Check sheet for the modelled part. Datum: model origin and axes. Units: mm. Face numbers are marked on the shaded views. A direction names the side the tool comes from. Round coordinates to 2 decimals unless told otherwise and drop trailing zeros. Loops run counter-clockwise (first coordinate to the right, second up) from the corner with the lowest first, then second, coordinate; pieces in that order, holes last. Notation, with made-up numbers: (73, 13) -> (96, 13) arc R32 cw to (96, 43) -> close; hole circle Ø7 at (-33, -29). An arc over 180 degrees is marked (long way). One line per item, written item: value. Start each with the question number.
1. Release check for a two-part mould opening along X. For the marked faces 1, 2 and 3 record: +X half, -X half, draft (parallel to the pull), parting line (faces both ways), or undercut.
2. Set-up check for the marked faces 4, 5, 6 and 7: record each of +Z, -Z, +X, -X, +Y, -Y from which the full face is reachable in a straight line by a thin tool's end or side.
3. Material ranges on L1, parallel to Y at x = 7, z = 19.5; L2, parallel to X at y = -1.5, z = 21; L3, parallel to Z at x = -14, y = 9.5, recorded low to high.
4. Go/stop test with flat-tipped pins: pin 1 (2.5 mm diameter, centred on y = 2.5, z = -6.5, fed in from -X); pin 2 (10 mm diameter, centred on x = 17.5, y = 3.5, fed in from +Z); pin 3 (11 mm diameter, centred on y = -5, z = -17.5, fed in from +X). Record where each tip stops, or that it passes through.
5. Cross-section at B-B on y = -25. Record the cut outline in (x, z).
6. Cross-section at A-A on x = 0. Record the cut outline in (y, z), then the cut area to 3 significant figures.
7. Cross-section at C-C on y = 6. Count the separate pieces of the cut face and the enclosed holes in it, then the cut area to 3 significant figures.
from build123d import *
from build123d.topology import SkipClean

# Parameters (mm, degrees)
HINGE_DEPTH           = 8.89
HINGE_2_DEPTH         = 8.89
SKETCH2_R             = 2.54
HINGE_HOLES_DEPTH     = 50.270844447
BODY_START            = 12.7
BODY_DEPTH            = 12.7
BOTTOM_PLATE_START    = 5.08
BOTTOM_PLATE_DEPTH    = 5.08
TUBE_CONNECTION_DEPTH = 19.05
BACKSTOP_DEPTH        = 2.921
CONNECT_TO_BASE_START = 12.7
CONNECT_TO_BASE_DEPTH = 12.7
SKETCH13_R            = 7.62
BOLT_ACCESS_DEPTH     = 21.59
BOTTOM_CHAMFER_SIZE   = 1.27


with BuildPart() as part:
    # Sketch1 → hinge (new body)
    with BuildSketch(Plane(origin=(0, 0, 0), x_dir=(1, 0, 0), z_dir=(0, 1, 0))):
        with BuildLine():
            ThreePointArc((-6.35, 26.882708313), (-9.597376484, 25.901599774), (-12.7, 24.529828908))
            Line((-12.7, 24.529828908), (-12.7, 11.829828908))
            Line((-12.7, 11.829828908), (-24.961122857, 11.829828908))
            ThreePointArc((-24.961122857, 11.829828908), (-26.9489436, 6.062750619), (-27.6225, 0))
            Line((-27.6225, 0), (-25.0825, 0))
            ThreePointArc((-25.0825, 0), (-24.632521559, 4.729766155), (-23.298731406, 9.289828908))
            Line((-23.298731406, 9.289828908), (-12.7, 9.289828908))
            Line((-12.7, 9.289828908), (-12.7, 0))
            Line((-12.7, 0), (-6.35, 0))
            Line((-6.35, 0), (-6.35, 26.882708313))
        make_face()
    hinge = extrude(amount=HINGE_DEPTH)


with BuildPart() as body_2:
    # Sketch1 → hinge 2 (new body)
    with BuildSketch(Plane(origin=(0, 0, 0), x_dir=(1, 0, 0), z_dir=(0, 1, 0))):
        with BuildLine():
            ThreePointArc((12.7, 24.529828908), (9.597376484, 25.901599774), (6.35, 26.882708313))
            Line((6.35, 26.882708313), (6.35, 0))
            Line((6.35, 0), (12.7, 0))
            Line((12.7, 0), (12.7, 9.289828908))
            Line((12.7, 9.289828908), (23.298731406, 9.289828908))
            ThreePointArc((23.298731406, 9.289828908), (24.632521559, 4.729766155), (25.0825, 0))
            Line((25.0825, 0), (27.6225, 0))
            ThreePointArc((27.6225, 0), (26.9489436, 6.062750619), (24.961122857, 11.829828908))
            Line((24.961122857, 11.829828908), (12.7, 11.829828908))
            Line((12.7, 11.829828908), (12.7, 24.529828908))
        make_face()
    hinge_2 = extrude(amount=HINGE_2_DEPTH)


with BuildPart() as hinge_holes_tool:
    # Sketch2 → hinge_holes (new, through all)
    with BuildSketch(Plane(origin=(12.7, 0, 0), x_dir=(0, 0, -1), z_dir=(1, 0, 0))):
        with Locations((19.262708313, 4.445)):
            Circle(SKETCH2_R)
    hinge_holes = extrude(amount=-HINGE_HOLES_DEPTH)


with BuildPart() as part_1:
    add(part.part)

    # hinge_holes: cut by hinge_holes_tool
    add(hinge_holes_tool.part, mode=Mode.SUBTRACT)



with BuildPart() as body_2_1:
    add(body_2.part)

    # hinge_holes: cut by hinge_holes_tool
    add(hinge_holes_tool.part, mode=Mode.SUBTRACT)


with BuildPart() as part_2:
    add(part_1.part)

    add(body_2_1.part)  # body merges body 2
    # Sketch5 → body (add)
    with BuildSketch(Plane.XZ.offset(BODY_START)):
        with BuildLine():
            Line((-27.6225, 0), (-25.0825, 0))
            ThreePointArc((-25.0825, 0), (-19.854542065, -15.327392656), (-6.35, -24.265393181))
            Line((-6.35, -24.265393181), (-6.35, -26.882708313))
            ThreePointArc((-6.35, -26.882708313), (-21.661087014, -17.140589711), (-27.6225, 0))
        make_face()
        with BuildLine():
            Line((25.0825, 0), (27.6225, 0))
            ThreePointArc((27.6225, 0), (21.661087014, -17.140589711), (6.35, -26.882708313))
            Line((6.35, -26.882708313), (6.35, -24.265393181))
            ThreePointArc((6.35, -24.265393181), (19.854542065, -15.327392656), (25.0825, 0))
        make_face()
    body = extrude(amount=-BODY_DEPTH)

    # Sketch6 → bottom_plate (add)
    with SkipClean():  # the faces are left unmerged after this step: merging them gives an invalid solid
        with BuildSketch(Plane.XZ.offset(12.7).offset(BOTTOM_PLATE_START)):
            with BuildLine():
                Line((13.97, 0), (3.81, 0))
                ThreePointArc((3.81, 0), (0, -3.81), (-3.81, 0))
                Line((-3.81, 0), (-13.97, 0))
                ThreePointArc((-13.97, 0), (-17.78, -3.81), (-21.59, 0))
                Line((-21.59, 0), (-27.6225, 0))
                ThreePointArc((-27.6225, 0), (0, -27.6225), (27.6225, 0))
                Line((27.6225, 0), (21.59, 0))
                ThreePointArc((21.59, 0), (17.78, -3.81), (13.97, 0))
            make_face()
        bottom_plate = extrude(amount=-BOTTOM_PLATE_DEPTH)

    # Sketch7 → tube_connection (add)
    with SkipClean():  # the faces are left unmerged after this step: merging them gives an invalid solid
        with BuildSketch(Plane.XZ.offset(17.78)):
            with BuildLine():
                Line((-22.86, 0), (-25.4, 0))
                ThreePointArc((-25.4, 0), (0, -25.4), (25.4, 0))
                Line((25.4, 0), (22.86, 0))
                ThreePointArc((22.86, 0), (0, -22.86), (-22.86, 0))
            make_face()
        tube_connection = extrude(amount=TUBE_CONNECTION_DEPTH)

    # Sketch10 → backstop (add)
    with SkipClean():  # the faces are left unmerged after this step: merging them gives an invalid solid
        with BuildSketch(Plane(origin=(0, 8.89, 0), x_dir=(1, 0, 0), z_dir=(0, 1, 0))):
            with BuildLine():
                Line((-23.298731406, 9.289828908), (-6.35, 9.289828908))
                Line((-6.35, 9.289828908), (-6.35, 11.829828908))
                Line((-6.35, 11.829828908), (-24.961122857, 11.829828908))
                ThreePointArc((-24.961122857, 11.829828908), (-26.9489436, 6.062750619), (-27.6225, 0))
                Line((-27.6225, 0), (-25.0825, 0))
                ThreePointArc((-25.0825, 0), (-24.632521559, 4.729766155), (-23.298731406, 9.289828908))
            make_face()
            with BuildLine():
                Line((6.35, 11.829828908), (24.961122857, 11.829828908))
                ThreePointArc((24.961122857, 11.829828908), (26.9489436, 6.062750619), (27.6225, 0))
                Line((27.6225, 0), (25.0825, 0))
                ThreePointArc((25.0825, 0), (24.632521559, 4.729766155), (23.298731406, 9.289828908))
                Line((23.298731406, 9.289828908), (6.35, 9.289828908))
                Line((6.35, 9.289828908), (6.35, 11.829828908))
            make_face()
        backstop = extrude(amount=BACKSTOP_DEPTH)

    # Mirror1: hinge, hinge 2, hinge_holes, body, bottom_plate, tube_connection, backstop across plane
    with SkipClean():  # the faces are left unmerged after this step: merging them gives an invalid solid
        add(hinge.mirror(Plane(origin=(0, 8.89, 0), x_dir=(1, 0, 0), z_dir=(0, 0, 1))))
        add(hinge_2.mirror(Plane(origin=(0, 8.89, 0), x_dir=(1, 0, 0), z_dir=(0, 0, 1))))
        add(hinge_holes.mirror(Plane(origin=(0, 8.89, 0), x_dir=(1, 0, 0), z_dir=(0, 0, 1))), mode=Mode.SUBTRACT)
        add(body.mirror(Plane(origin=(0, 8.89, 0), x_dir=(1, 0, 0), z_dir=(0, 0, 1))))
        add(bottom_plate.mirror(Plane(origin=(0, 8.89, 0), x_dir=(1, 0, 0), z_dir=(0, 0, 1))))
        add(tube_connection.mirror(Plane(origin=(0, 8.89, 0), x_dir=(1, 0, 0), z_dir=(0, 0, 1))))
        add(backstop.mirror(Plane(origin=(0, 8.89, 0), x_dir=(1, 0, 0), z_dir=(0, 0, 1))))

    # Sketch12 → connect_to_base (add)
    with SkipClean():  # the faces are left unmerged after this step: merging them gives an invalid solid
        with BuildSketch(Plane.XZ.offset(CONNECT_TO_BASE_START)):
            with BuildLine():
                Line((-6.35, -24.265393181), (-6.35, 24.265393181))
                ThreePointArc((-6.35, 24.265393181), (-9.615737574, 23.166126071), (-12.7, 21.629651089))
                Line((-12.7, 21.629651089), (-12.7, 11.829828908))
                Line((-12.7, 11.829828908), (-22.117571165, 11.829828908))
                ThreePointArc((-22.117571165, 11.829828908), (-22.743637238, 10.576330717), (-23.298731406, 9.289828908))
                Line((-23.298731406, 9.289828908), (-12.7, 9.289828908))
                Line((-12.7, 9.289828908), (-12.7, -9.289828908))
                Line((-12.7, -9.289828908), (-23.298731406, -9.289828908))
                ThreePointArc((-23.298731406, -9.289828908), (-22.743637238, -10.576330717), (-22.117571165, -11.829828908))
                Line((-22.117571165, -11.829828908), (-12.7, -11.829828908))
                Line((-12.7, -11.829828908), (-12.7, -21.629651089))
                ThreePointArc((-12.7, -21.629651089), (-9.615737574, -23.166126071), (-6.35, -24.265393181))
            make_face()
            with BuildLine():
                Line((12.7, 9.289828908), (23.298731406, 9.289828908))
                ThreePointArc((23.298731406, 9.289828908), (22.743637238, 10.576330717), (22.117571165, 11.829828908))
                Line((22.117571165, 11.829828908), (12.7, 11.829828908))
                Line((12.7, 11.829828908), (12.7, 21.629651089))
                ThreePointArc((12.7, 21.629651089), (9.615737574, 23.166126071), (6.35, 24.265393181))
                Line((6.35, 24.265393181), (6.35, -24.265393181))
                ThreePointArc((6.35, -24.265393181), (9.615737574, -23.166126071), (12.7, -21.629651089))
                Line((12.7, -21.629651089), (12.7, -11.829828908))
                Line((12.7, -11.829828908), (22.117571165, -11.829828908))
                ThreePointArc((22.117571165, -11.829828908), (22.743637238, -10.576330717), (23.298731406, -9.289828908))
                Line((23.298731406, -9.289828908), (12.7, -9.289828908))
                Line((12.7, -9.289828908), (12.7, 9.289828908))
            make_face()
        extrude(amount=-CONNECT_TO_BASE_DEPTH)
    add(part_2.part.scale(1), mode=Mode.REPLACE)  # the faces are merged on a copy

    # Sketch13 → bolt_access (cut)
    with BuildSketch(Plane(origin=(0, -12.7, 0), x_dir=(1, 0, 0), z_dir=(0, 1, 0))):
        Circle(SKETCH13_R)
    extrude(amount=BOLT_ACCESS_DEPTH, mode=Mode.SUBTRACT)

    # bottom_chamfer
    bottom_chamfer_edges = [part_2.edges().sort_by_distance(p)[0] for p in [
        (0, -36.83, -25.4),
    ]]
    chamfer(bottom_chamfer_edges, length=BOTTOM_CHAMFER_SIZE)


solid = part_2.part
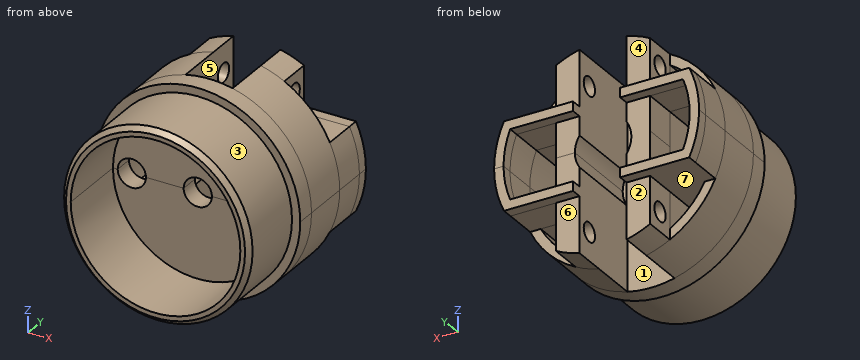
Taken from the geometry:
1. face 1: undercut
1. face 2: draft
1. face 3: parting line
2. face 4: +Z, +X, -X, +Y
2. face 5: +Z, -Z, +Y
2. face 6: -Z, +X, -X, +Y
2. face 7: +Y
3. L1: y = -17.78 to 1.92, 6.97 to 8.89
3. L2: x = -17.94 to -13.72, -12.7 to -6.35, 6.35 to 12.7, 13.72 to 17.94
3. L3: z = -11.83 to -9.29, 9.29 to 11.83
4. pin 1: stops at x = -27.12
4. pin 2: stops at z = 24.63
4. pin 3: stops at x = 24.88
5. outline: circle Ø50.8 at (0, 0); hole circle Ø45.72 at (0, 0)
6. outline: (-36.83, -24.13) -> (-35.56, -25.4) -> (-17.78, -25.4) -> (-17.78, -27.62) -> (-12.7, -27.62) -> (-12.7, -3.81) -> (-17.78, -3.81) -> (-17.78, -22.86) -> (-36.83, -22.86) -> close; (-36.83, 22.86) -> (-17.78, 22.86) -> (-17.78, 3.81) -> (-12.7, 3.81) -> (-12.7, 27.62) -> (-17.78, 27.62) -> (-17.78, 25.4) -> (-35.56, 25.4) -> (-36.83, 24.13) -> close
6. area: 337 mm2
7. separate pieces: 6
7. enclosed holes: 2
7. area: 767 mm2
